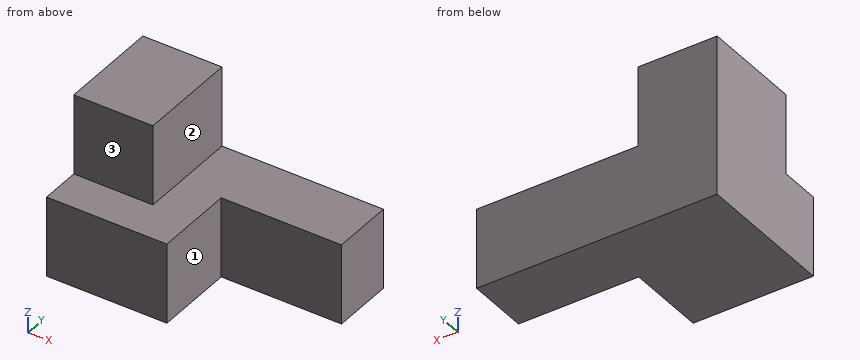
```python
from build123d import *

# Parameters (mm, degrees)
F0_W     = 25.075742
F0_H     = 25.4
F0_W_2   = 38.1
F3_DEPTH = 44.98379
F1_W     = 12.7
F1_H     = 25.4
F4_DEPTH = 25.60555
F5_DEPTH = 25.4


with BuildPart() as f3:
    # F0 (on Front) → F3 (new body)
    with BuildSketch(Plane.XZ):
        Polygon((0, 25.4), (0, 0), (38.1, 0), (38.1, 25.4), (25.075742, 25.4), align=None)
        with Locations((12.537871, 38.1)):
            Rectangle(F0_W, F0_H)
        with Locations((57.15, 12.7)):
            Rectangle(F0_W_2, F0_H)
    extrude(amount=-F3_DEPTH)

    # F1 (on Right) → F4 (cut)
    with BuildSketch(Plane.YZ):
        with Locations((6.35, 38.1)):
            Rectangle(F1_W, F1_H)
    extrude(amount=F4_DEPTH, mode=Mode.SUBTRACT)

    # F2 (on Top) → F5 (cut)
    with BuildSketch(Plane.XY):
        Polygon((76.496184, 0), (76.2, 25.4), (38.1, 25.4), (38.1, 0), align=None)
    extrude(amount=F5_DEPTH, mode=Mode.SUBTRACT)


solid = f3.part
```
The listing builds one solid part. Answer for the finished solid, in the listing's coordinates (mm). Face numbers are marked on the shaded views. A direction names the side the tool comes from. Coordinates: 2 decimals unless noted, no trailing zeros. Write each loop counter-clockwise with the first axis right and the second up, starting at its lowest first coordinate (ties: lowest second). Pieces come first, ordered by that corner, then holes. Notation, with made-up numbers: (-12, -16) - (40, -16) arc R21 ccw to (40, 18) - close; hole circle Ø6 at (41.5, 27). An arc over 180 degrees is marked (long way). One line per item, written item: value.
1) Each of these flat-tipped pins is pushed along its axis until it touches: pin 1 Ø10 at (y, z) = (9, 6) entering from +X; pin 2 Ø12.5 at (x, z) = (10.5, 33.5) entering from -Y; pin 3 Ø7.5 at (y, z) = (29.5, 37.5) entering from +X. Where does it stop, or does it pass through?
Geometry check:
pin 1: stops at x = 38.1
pin 2: stops at y = 12.7
pin 3: stops at x = 25.08
2) A tool of negligible diameter and unlimited length cuts with its end or side. For the marked faces 1, 2 and 3, from which of +Z, -Z, +X, -X, +Y, -Y can it reach the whole face along a straight path? Write none if from no direction.
Geometry check:
face 1: +Z, -Z, +X, -Y
face 2: +Z, +X, +Y, -Y
face 3: +Z, +X, -X, -Y
3) Consider line 1 along X through (y, z) = (31.5, 37.5); line 2 along Z through (x, y) = (37.5, 14); line 3 along Y through (x, z) = (11.5, 43). Determine where each line is inside the solid, lowest interval first. Write a range as from..to.
Geometry check:
line 1: x = 0..25.08
line 2: z = 0..25.4
line 3: y = 12.7..44.98
4) Find section B-B (x = 23.5). Give the vertices of the cut face in (y, z), and give its area (3 significant figures).
Geometry check:
outline: (0, 0) - (44.98, 0) - (44.98, 50.8) - (12.7, 50.8) - (12.7, 25.4) - (0, 25.4) - close
area: 1,960 mm2
5) Find section A-A (y = 19.5). Give the vertices of the cut face in (x, z).
Geometry check:
outline: (0, 0) - (38.1, 0) - (38.1, 25.4) - (25.08, 25.4) - (25.08, 50.8) - (0, 50.8) - close
6) Find section D-D (x = 36). Give the vertices of the cut face in (y, z).
Geometry check:
outline: (0, 0) - (44.98, 0) - (44.98, 25.4) - (0, 25.4) - close
7) Find section C-C (z = 38). Give the vertices of the cut face in (x, y).
Geometry check:
outline: (0, 12.7) - (25.08, 12.7) - (25.08, 44.98) - (0, 44.98) - close
